Autodesk Inventor part; units mm, degrees
ref_plane "YZ Plane" through (0, 0, 0) normal (1, 0, 0) x (0, 1, 0)
ref_plane "XZ Plane" through (0, 0, 0) normal (0, 1, 0) x (-1, 0, 0)
ref_plane "XY Plane" through (0, 0, 0) normal (0, 0, 1) x (1, 0, 0)
sketch "Náčrt1" plane through (0, 0, 0) normal (0, 1, 0) x (-1, 0, 0)
  line L0 (75, 75) -> (-75, 75)
  line L1 (-75, 75) -> (-75, -75)
  line L2 (-75, -75) -> (75, -75)
  line L3 (75, -75) -> (75, 75)
  line L4 (75, 75) -> (-75, -75) construction
  line L5 (-75, 75) -> (75, -75) construction
  point P0 (0, 0)
  dimension "d0" = 150
  dimension "d1" = 150
extrude "Vysunutí1" add sketch "Náčrt1" along normal blind 30
sketch "Náčrt2" plane through (0, 30, 0) normal (0, 1, 0) x (1, 0, 0)
  line L0 (75, -75) -> (-75, -75)
  line L1 (-75, -75) -> (-75, 75)
  line L2 (-75, 75) -> (75, 75)
  line L3 (75, 75) -> (75, -75)
  line L4 (75, -75) -> (-75, 75) construction
  line L5 (-75, -75) -> (75, 75) construction
  line L6 (45, -45) -> (-45, -45)
  line L7 (-45, -45) -> (-45, 45)
  line L8 (-45, 45) -> (45, 45)
  line L9 (45, 45) -> (45, -45)
  line L10 (45, -45) -> (-45, 45) construction
  line L11 (-45, -45) -> (45, 45) construction
  point P0 (0, 0)
  dimension "d4" = 150
  dimension "d5" = 150
  dimension "d6" = 90
  dimension "d7" = 90
extrude "Vysunutí2" add sketch "Náčrt2" along normal blind 90
sketch "Náčrt3" plane through (-75, 0, 75) normal (0, 0, 1) x (1, 0, 0)
  line L0 (120, 30) -> (30, 30)
  line L1 (60, 30) -> (90, 30)
  line L2 (90, 30) -> (90, 90)
  line L3 (90, 90) -> (60, 90)
  line L4 (60, 90) -> (60, 30)
  point P0 (75, 0)
  dimension "d10" = 30
  dimension "d11" = 60
extrude "Vysunutí3" cut sketch "Náčrt3" against normal blind 90
sketch "Náčrt4" plane through (75, 0, 75) normal (1, 0, 0) x (0, 0, -1)
  line L0 (60, 60) -> (90, 60)
  line L1 (90, 60) -> (90, 90)
  line L2 (90, 90) -> (60, 90)
  line L3 (60, 90) -> (60, 60)
  point P0 (75, 0)
  dimension "d14" = 30
  dimension "d15" = 30
extrude "Vysunutí4" cut sketch "Náčrt4" against normal through all
sketch "Náčrt5" plane through (75, 0, -75) normal (0, 0, -1) x (-1, 0, 0)
  line L0 (60, 30) -> (60, 90)
  line L1 (60, 90) -> (90, 90)
  line L2 (90, 90) -> (90, 60)
  line L3 (90, 60) -> (60, 60)
  line L4 (60, 60) -> (60, 90)
  point P0 (75, 0)
  dimension "d18" = 30
  dimension "d19" = 30
extrude "Vysunutí5" cut sketch "Náčrt5" against normal through all
sketch "Náčrt6" plane through (0, 0, 0) normal (1, 0, 0) x (0, 1, 0)
  line L0 (0, 75) -> (120, 75)
  line L1 (0, 75) -> (0, -75)
  line L2 (0, 75) -> (30, 75)
  line L3 (30, 75) -> (30, 105)
  line L4 (30, 105) -> (0, 105)
  line L5 (0, 105) -> (0, 75)
  line L6 (30, 105) -> (15, 105)
  line L7 (15, 105) -> (15, 90)
  line L8 (15, 90) -> (30, 90)
  line L9 (30, 90) -> (30, 105)
  point P0 (0, 0)
  dimension "d28" = 30
  dimension "d29" = 30
  dimension "d30" = 15
  dimension "d31" = 15
extrude "Vysunutí6" add sketch "Náčrt6" along normal mid plane 90 contours L5 L4 L7 L8 L3 L0
sketch "Náčrt7" plane through (0, 120, 0) normal (0, 1, 0) x (1, 0, 0)
  line L0 (15, -45) -> (45, -45)
  line L1 (-45, 45) -> (45, 45)
  line L2 (45, 45) -> (45, -45)
  line L3 (45, -45) -> (-45, -45)
  line L4 (-45, -45) -> (-45, 45)
  line L5 (-45, 45) -> (45, -45) construction
  line L6 (45, 45) -> (-45, -45) construction
  line L7 (-55, 55) -> (55, 55)
  line L8 (55, 55) -> (55, -55)
  line L9 (55, -55) -> (-55, -55)
  line L10 (-55, -55) -> (-55, 55)
  line L11 (-55, 55) -> (55, -55) construction
  line L12 (55, 55) -> (-55, -55) construction
  point P0 (0, 0)
  dimension "d32" = 110
  dimension "d33" = 110
extrude "Vysunutí7" add sketch "Náčrt7" along normal blind 10
sketch "Náčrt9" plane through (0, 0, 0) normal (0, -1, 0) x (1, 0, 0)
  line L0 (75, 75) -> (75, -75)
  line L1 (-75, 75) -> (-45, 75)
  point P0 (0, 0)
  point P1 (60, 60)
  point P2 (60, -60)
  point P3 (-60, -60)
  point P4 (-60, 60)
  dimension "d48" = 120
  dimension "d49" = 120
  dimension "d50" = 15
  dimension "d58" = 15
hole "Díra1" at (60, 0, 60) at (60, 0, -60) at (-60, 0, -60) at (-60, 0, 60) direction (0, 1, 0) diameter 2 depth 8 tip angle 118
sketch "Náčrt10" plane through (0, 120, 0) normal (0, 1, 0) x (1, 0, 0)
  line L0 (61, -20) -> (59, -20)
  line L1 (59, -20) -> (59, 20)
  line L2 (59, 20) -> (61, 20)
  line L3 (61, 20) -> (61, -20)
  line L4 (75, -75) -> (75, 75)
  line L5 (45, 45) -> (45, -45)
  line L6 (75, 15) -> (45, 15)
  line L7 (75, -15) -> (45, -15)
  line L8 (0, 17.5556) -> (0, -18.0256) construction
  line L9 (-61, -20) -> (-59, -20)
  line L10 (-59, -20) -> (-59, 20)
  line L11 (-59, 20) -> (-61, 20)
  line L12 (-61, 20) -> (-61, -20)
  line L13 (-75, 15) -> (-45, 15)
  line L14 (-75, -15) -> (-45, -15)
  line L15 (75, 75) -> (-75, 75) construction
  line L16 (0, 0) -> (-75, 75) construction
  line L17 (20, 61) -> (20, 59)
  line L18 (20, 59) -> (-20, 59)
  line L19 (-20, 59) -> (-20, 61)
  line L20 (-20, 61) -> (20, 61)
  line L21 (-15, 75) -> (-15, 45)
  line L22 (15, 75) -> (15, 45)
  point P0 (59, 0)
  point P1 (60, 20)
  point P2 (60, -20)
  point P3 (-59, 0)
  point P4 (-60, 20)
  point P5 (-60, -20)
  point P6 (0, 59)
  point P7 (-20, 60)
  point P8 (20, 60)
  dimension "d51" = 2
  dimension "d52" = 14
  dimension "d53" = 14
  dimension "d54" = 5
  dimension "d55" = 5
extrude "Vysunutí9" cut sketch "Náčrt10" against normal blind 60 contours L0 L1 L7 L3 | L7 L1 L6 L3 | L6 L1 L2 L3 | L12 L14 L10 L9 | L12 L13 L10 L14 | L12 L11 L10 L13 | L17 L18 L22 L20 | L22 L18 L21 L20 | L21 L18 L19 L20
sketch "Náčrt11" plane through (0, 0, 0) normal (0, -1, 0) x (1, 0, 0)
  line L0 (-75, 75) -> (-45, 75)
  line L1 (10.5, 78.25) -> (-23.5, 78.25)
  line L2 (-23.5, 78.25) -> (-23.5, 65.75)
  line L3 (-23.5, 65.75) -> (10.5, 65.75)
  line L4 (10.5, 65.75) -> (10.5, 78.25)
  line L5 (-45, 75) -> (-45, 105)
  circle A0 centre (-12, 72) radius 6.25
  point P0 (0, 0)
  point P1 (-23.5, 72)
  dimension "d65" = 34
  dimension "d66" = 12.5
  dimension "d92" = 11.5
extrude "Vysunutí10" cut sketch "Náčrt11" against normal blind 21
sketch "Náčrt13" plane through (0, 21, 0) normal (0, -1, 0) x (1, 0, 0)
  line L0 (10.5, 65.75) -> (-23.5, 65.75)
  line L1 (-23.5, 78.25) -> (10.5, 78.25)
  line L2 (-19, 65.75) -> (5, 65.75)
  line L3 (5, 65.75) -> (5, 78.25)
  line L4 (5, 78.25) -> (-19, 78.25)
  line L5 (-19, 78.25) -> (-19, 65.75)
  line L6 (10.5, 78.25) -> (10.5, 65.75)
  line L7 (-23.5, 65.75) -> (-23.5, 78.25)
  point P0 (0, 0)
  point P1 (-15, 78.25)
  point P2 (10.5, 72)
  point P3 (5, 72)
  point P4 (-23.5, 75)
  point P5 (-19, 72)
  dimension "d79" = 24
  dimension "d80" = 5.5
  dimension "d81" = 4.5
extrude "Vysunutí12" cut sketch "Náčrt13" against normal blind 4.5 contours L0 L5 L1 L3
sketch "Náčrt15" plane through (-75, 120, 75) normal (0, 0, 1) x (1, 0, 0)
  line L0 (95.25, -41.75) -> (114.75, -41.75)
  line L1 (114.75, -41.75) -> (114.75, -48.25)
  line L2 (114.75, -48.25) -> (95.25, -48.25)
  line L3 (95.25, -48.25) -> (95.25, -41.75)
  line L4 (60, -30) -> (90, -30)
  line L5 (90, -30) -> (120, -30)
  line L6 (120, -30) -> (120, -60)
  line L7 (120, -60) -> (90, -60)
  line L8 (90, -60) -> (90, -30)
  point P0 (75, -120)
  point P1 (105, -41.75)
  point P2 (114.75, -45)
  dimension "d95" = 30
  dimension "d96" = 6.5
  dimension "d97" = 19.5
  dimension "d98" = 15
  dimension "d99" = 15
  dimension "d100" = 15
extrude "Vysunutí14" cut sketch "Náčrt15" against normal blind 20 contours L0 L1 L2 L3
sketch "Náčrt16" plane through (0, 0, 0) normal (0, -1, 0) x (1, 0, 0)
  line L0 (20.25, 75) -> (20.25, 55)
  line L1 (39.75, 75) -> (39.75, 55)
  line L2 (20.25, 72) -> (39.75, 72)
  line L3 (39.75, 72) -> (39.75, 55)
  line L4 (39.75, 55) -> (20.25, 55)
  line L5 (20.25, 55) -> (20.25, 72)
  line L6 (45, 75) -> (75, 75)
  point P0 (0, 0)
  dimension "d103" = 17
  dimension "d104" = 3
extrude "Vysunutí15" cut sketch "Náčrt16" against normal through all
sketch "Náčrt17" plane through (-45, 15, 90) normal (0, 0, 1) x (1, 0, 0)
  line L0 (90, 15) -> (75, 15)
  line L1 (75, 15) -> (75, 0)
  line L2 (75, 0) -> (90, 0)
  line L3 (90, 0) -> (90, 15)
  line L4 (0, 15) -> (30, 15)
  line L5 (0, 15) -> (15, 15)
  line L6 (15, 15) -> (15, 0)
  line L7 (15, 0) -> (0, 0)
  line L8 (0, 0) -> (0, 15)
  point P0 (45, -15)
  dimension "d107" = 15
  dimension "d108" = 15
  dimension "d109" = 15
  dimension "d110" = 15
extrude "Vysunutí16" cut sketch "Náčrt17" against normal blind 15
sketch "Náčrt18" plane through (0, 25.5, 0) normal (0, -1, 0) x (1, 0, 0)
  circle A0 centre (-12, 72) radius 6.25
  line L0 (-23.5, 78.25) -> (10.5, 78.25)
  line L1 (-23.5, 65.75) -> (-23.5, 78.25)
  circle A1 centre (-5.75, 72) radius 3
  point P0 (0, 0)
  point P1 (-6.47, 69.0877)
  point P2 (-6.47, 74.9123)
  dimension "d114" = 12.5
  dimension "d113" = 11.5
  dimension "d115" = 6
extrude "Vysunutí17" cut sketch "Náčrt18" against normal blind 4.5
sketch "Náčrt19" plane through (0, 120, 0) normal (0, 1, 0) x (1, 0, 0)
  arc A0 (-17.4829, -75) -> (-6.47, -74.9123) centre (-12, -72) ccw
  circle A1 centre (-12, -72) radius 0.5
  point P0 (0, 0)
  dimension "d118" = 1
extrude "Vysunutí18" cut sketch "Náčrt19" against normal blind 30
sketch "Náčrt20" plane through (0, 120, 0) normal (0, 1, 0) x (1, 0, 0)
  line L0 (39.75, -55) -> (39.75, -72)
  line L1 (39.75, -55) -> (49.75, -55)
  line L2 (49.75, -55) -> (49.75, -65)
  line L3 (49.75, -65) -> (39.75, -65)
  line L4 (39.75, -65) -> (39.75, -55)
  point P0 (0, 0)
  dimension "d121" = 10
  dimension "d122" = 10
extrude "Vysunutí19" cut sketch "Náčrt20" against normal through all
properties part number "steny" material "Beton"
Geometry check sheet. Reference: the model listing, model coordinates, mm. A direction names the side the tool comes from. Coordinates: 2 decimals unless noted, no trailing zeros. Order: outer loops, then holes, each group sorted by start corner. A loop starts at its lowest first (then second) coordinate and runs counter-clockwise, first axis right, second up. Notation, with made-up numbers: (52, 80) - (92, 80) arc R16 ccw to (92, 96) - close; hole circle Ø7 at (77.5, 73.25). An arc over 180 degrees is marked (long way). Answer in a Markdown table with one row per item. Add a question column.
1) Gauge pin test, flat ends, axial feed: P1, Ø7.5, axis at x = -12, z = 72, coming from the +Y side; P2, Ø6, axis at x = -24, y = 23, coming from the +Z side; P3, Ø12, axis at x = 53, y = 15, coming from the +Z side. Record the tip position at first contact, or that the pin passes through.
2) Cross-section at C-C, the plane x = -27.5. Record the cut outline in (y, z), then the cut area to 3 significant figures.
3) Material ranges on line 1 along Z through (x, y) = (39, 65); line 2 along X through (y, z) = (43, 69); line 3 along Z through (x, y) = (-9.5, 90.5), recorded low to high. Write a range as [from, to].
4) Release check for a two-part mould opening along Y. For faces 4 (the flat face through (30, 99, 72)), 5 (the flat face through (68, 90, 0)), 6 (the flat face through (-18.4, 25.5, 71.6)) record: +Y half, -Y half, draft (parallel to the pull), parting line (faces both ways), or undercut.
5) Set-up check for faces 1 (the flat face through (52, 75, -15)), 2 (the flat face through (-15, 75, -68)), 3 (the flat face through (25, 79, 55)): record each of +Z, -Z, +X, -X, +Y, -Y from which the full face is reachable in a straight line by a thin tool's end or side.
6) Cross-section at A-A, the plane y = 102. Record the cut outline in (x, z).
7) Cross-section at D-D, the plane z = 35. Record the cut outline in (x, y), then the cut area to 3 significant figures.
8) Cross-section at B-B, the plane z = -9.5. Record the cut outline in (x, y), then the cut area to 3 significant figures.
Check result:
| question | item | result |
|---|---|---|
| 1 | P1 | stops at y = 120 |
| 1 | P2 | stops at z = 90 |
| 1 | P3 | stops at z = 75 |
| 2 | outline | (0, -75) - (120, -75) - (120, -55) - (130, -55) - (130, -45) - (30, -45) - (30, 45) - (130, 45) - (130, 55) - (120, 55) - (120, 75) - (30, 75) - (30, 90) - (15, 90) - (15, 105) - (0, 105) - close |
| 2 | area | 10,800 mm² |
| 3 | line 1 | z = [-75, -45], [45, 55], [72, 75] |
| 3 | line 2 | x = [-75, -15], [15, 20.25], [39.75, 75] |
| 3 | line 3 | z = [-75, -61], [-59, -45], [45, 75] |
| 4 | face 4 | draft |
| 4 | face 5 | undercut |
| 4 | face 6 | -Y half |
| 5 | face 1 | +X, -X |
| 5 | face 2 | +Z, -Z |
| 5 | face 3 | +Y |
| 6 | outline | (-75, -75) - (75, -75) - (75, 75) - (-75, 75) - close; hole (-61, -20) - (-59, -20) - (-59, 20) - (-61, 20) - close; hole (-45, -45) - (45, -45) - (45, 45) - (-45, 45) - close; hole (-20, -61) - (20, -61) - (20, -59) - (-20, -59) - close; hole circle Ø1 at (-12, 72); hole (20.25, 55) - (49.75, 55) - (49.75, 65) - (39.75, 65) - (39.75, 72) - (20.25, 72) - close; hole (59, -20) - (61, -20) - (61, 20) - (59, 20) - close |
| 7 | outline | (-75, 0) - (75, 0) - (75, 120) - (55, 120) - (55, 130) - (45, 130) - (45, 30) - (-45, 30) - (-45, 130) - (-55, 130) - (-55, 120) - (-75, 120) - close |
| 7 | area | 10,100 mm² |
| 8 | outline | (-75, 0) - (75, 0) - (75, 60) - (45, 60) - (45, 30) - (-45, 30) - (-45, 60) - (-75, 60) - close; (-75, 90) - (-61, 90) - (-61, 120) - (-75, 120) - close; (-59, 90) - (-45, 90) - (-45, 130) - (-55, 130) - (-55, 120) - (-59, 120) - close; (45, 90) - (59, 90) - (59, 120) - (55, 120) - (55, 130) - (45, 130) - close; (61, 90) - (75, 90) - (75, 120) - (61, 120) - close |
| 8 | area | 8,180 mm² |
